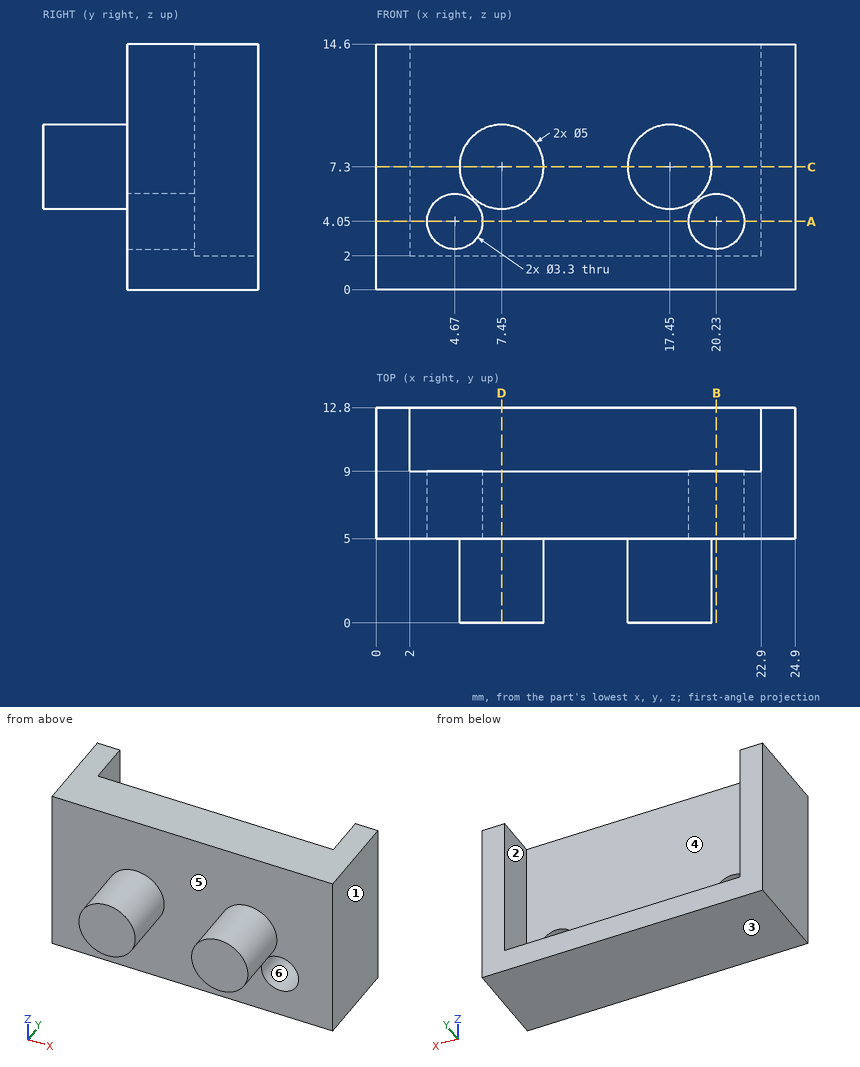
Verification items for this drawing (mm, ordinates from the low corner). A direction names the side the tool comes from. Give positions to 0.01 mm unless a question says otherwise; leave off trailing zeros. Loops run counter-clockwise (first coordinate to the right, second up) from the corner with the lowest first, then second, coordinate; pieces in that order, holes last. Notation, with made-up numbers: M 9,22.5 L 19,22.5 A21 cw 19,39.5 Z; hole C -11,17 d5. An arc over 180 degrees is marked long. Answer as a JSON object with one key per item and string values. Group by question number.
Item 1: Access from +Z, -Z, +X, -X, +Y, -Y to the whole of each face (thin tool, end or side, straight path). Record for the marked faces 4, 5 and 6.
Item 2: Material ranges on L1, parallel to X at y = 7.2, z = 4.05; L2, parallel to X at y = 9.75, z = 2.5; L3, parallel to X at y = 6.5, z = 4.75, recorded low to high.
Item 3: Sectioned sample at D-D on x = 7.45. Record the boundary of the cut face in (y, z), plus the area to 3 significant figures.
Item 4: Gauge pin test, flat ends, axial feed: pin 1 (3 mm diameter, centred on x = 18, z = 8, fed in from +Y); pin 2 (3 mm diameter, centred on x = 14, y = 10, fed in from +Z); pin 3 (1.5 mm diameter, centred on y = 4, z = 7.5, fed in from +X). Record the tip position at first contact, or that the pin passes through.
Item 5: Mould release check, pull along X, two halves, no side actions. Record for the marked faces 1, 2 and 3: pulls with the +X half, pulls with the -X half, needs draft (parallel to the pull), parting line crosses it, or undercut.
Item 6: Sectioned sample at B-B on x = 20.23. Record the boundary of the cut face in (y, z).
Item 7: Sectioned sample at C-C on z = 7.3. Record the boundary of the cut face in (x, y).
Item 8: Sectioned sample at A-A on z = 4.05. Record the boundary of the cut face in (x, y), plus the area to 3 significant figures.
Findings below:
{
 "1": {"face 4": "+Z, +Y", "face 5": "-Y", "face 6": "+Y, -Y"},
 "2": {"L1": "0 to 3.02, 6.32 to 18.58, 21.88 to 24.9", "L2": "0 to 2, 22.9 to 24.9", "L3": "0 to 3.18, 6.16 to 18.74, 21.72 to 24.9"},
 "3": {"outline": "M 0,4.8 L 5,4.8 L 5,0 L 12.8,0 L 12.8,2 L 9,2 L 9,14.6 L 5,14.6 L 5,9.8 L 0,9.8 Z", "area": "91.0 mm2"},
 "4": {"pin 1": "y = 9", "pin 2": "z = 14.6", "pin 3": "x = 19.95"},
 "5": {"face 1": "pulls with the +X half", "face 2": "undercut", "face 3": "needs draft"},
 "6": {"outline": "M 5,0 L 12.8,0 L 12.8,2 L 9,2 L 9,2.4 L 5,2.4 Z; M 5,5.7 L 9,5.7 L 9,14.6 L 5,14.6 Z"},
 "7": {"outline": "M 0,5 L 4.95,5 L 4.95,0 L 9.95,0 L 9.95,5 L 14.95,5 L 14.95,0 L 19.95,0 L 19.95,5 L 24.9,5 L 24.9,12.8 L 22.9,12.8 L 22.9,9 L 2,9 L 2,12.8 L 0,12.8 Z"},
 "8": {"outline": "M 0,5 L 3.02,5 L 3.02,9 L 2,9 L 2,12.8 L 0,12.8 Z; M 6.32,5 L 18.58,5 L 18.58,9 L 6.32,9 Z; M 21.88,5 L 24.9,5 L 24.9,12.8 L 22.9,12.8 L 22.9,9 L 21.88,9 Z", "area": "88.4 mm2"}
}
